Check sheet for the modelled part. Datum: model origin and axes. Units: mm. Face numbers are marked on the shaded views. A direction names the side the tool comes from. Round coordinates to 2 decimals unless told otherwise and drop trailing zeros. Order: outer loops, then holes, each group sorted by start corner. A loop starts at its lowest first (then second) coordinate and runs counter-clockwise, first axis right, second up. Notation, with made-up numbers: (34.5, 70) -> (80.5, 70) arc R9 ccw to (80.5, 77) -> close; hole circle Ø1 at (80.25, 73.25). An arc over 180 degrees is marked (long way). Answer in a Markdown table with one row per item.
```python
from build123d import *

# Parameters (mm, degrees)
F0_R     = 7.5
F1_DEPTH = 5
F2_R     = 6
F3_DEPTH = 1
F4_W     = 1.6
F4_H     = 1.2
F4_W_2   = 1.2
F4_H_2   = 1.6
F5_DEPTH = 3
F7_R     = 1.5


with BuildPart() as f1:
    # F0 (on Top) → F1 (new body)
    with BuildSketch(Plane.XY):
        Circle(F0_R)
    extrude(amount=F1_DEPTH)

    # F2 (on face) → F3 (join)
    with BuildSketch(Plane.XY.offset(5)):
        Circle(F2_R)
    extrude(amount=F3_DEPTH)

    # F4 (on face) → F5 (cut)
    with BuildSketch(Plane.XY.offset(6)):
        with Locations((0, 1.4)):
            Rectangle(F4_W, F4_H)
        with Locations((-1.4, 0)):
            Rectangle(F4_W_2, F4_H_2)
        Rectangle(F4_W, F4_H_2)
        with Locations((1.4, 0)):
            Rectangle(F4_W_2, F4_H_2)
        with Locations((0, -1.4)):
            Rectangle(F4_W, F4_H)
    extrude(amount=-F5_DEPTH, mode=Mode.SUBTRACT)

    # F7 (on Right) → F8 (revolve, cut)
    with BuildSketch(Plane.YZ):
        with Locations((-8, 2)):
            Circle(F7_R)
    revolve(axis=Axis((0, 0, 2.2380100563), (0, 0, -1)), mode=Mode.SUBTRACT)


solid = f1.part
```
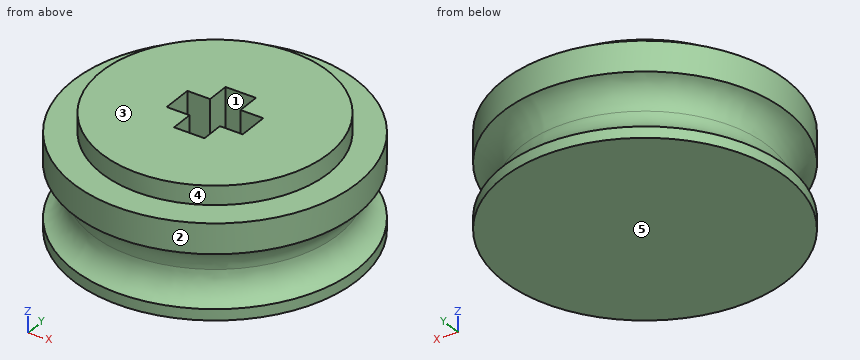
(1) Scan lines: probe 1 along X at (y, z) = (-1.25, 4.7); probe 2 along X at (y, z) = (0.75, 3.7); probe 3 along Z at (x, y) = (5.5, 3.25). Record each from-to range of solid material in increasing order. Write a range as from..to.
Solutions:
| item | result |
|---|---|
| probe 1 | -7.4..-0.8, 0.8..7.4 |
| probe 2 | -7.46..-2, 2..7.46 |
| probe 3 | 0..5 |
(2) Draft check along X on the marked faces 1, 2 and 3. Enter one of: pulls with the +X half, pulls with the -X half, needs draft (parallel to the pull), parting line crosses it, or undercut.
Solutions:
| item | result |
|---|---|
| face 1 | undercut |
| face 2 | parting line crosses it |
| face 3 | needs draft |
(3) Section check B-B on x = 0. Record the boundary of the cut face in (y, z).
Solutions:
| item | result |
|---|---|
| outline | (-7.5, 0) -> (7.5, 0) -> (7.5, 0.59) arc R1.5 cw to (7.5, 3.41) -> (7.5, 5) -> (6, 5) -> (6, 6) -> (2, 6) -> (2, 3) -> (-2, 3) -> (-2, 6) -> (-6, 6) -> (-6, 5) -> (-7.5, 5) -> (-7.5, 3.41) arc R1.5 cw to (-7.5, 0.59) -> close |
(4) Tool access check on the marked faces 4 and 5. Record the directions out of +Z, -Z, +X, -X, +Y, -Y that give a thin tool (end or side, any length) a straight path to the whole face; none if there is none.
Solutions:
| item | result |
|---|---|
| face 4 | +Z |
| face 5 | -Z, +X, -X, +Y, -Y |
(5) Depth check by flat-ended pin: pin 1 Ø1 at (x, z) = (1.5, 5) entering from -Y; pin 2 Ø3 at (y, z) = (2.5, 4.5) entering from +X; pin 3 Ø1 at (x, z) = (1.5, 4.5) entering from +Y. Enter the tip coordinate at first touch or a pass-through.
Solutions:
| item | result |
|---|---|
| pin 1 | y = -7.43 |
| pin 2 | x = 7.43 |
| pin 3 | y = 7.43 |
(6) Section check A-A on z = 4.25. Record the boundary of the cut face in (x, y).
Solutions:
| item | result |
|---|---|
| outline | circle Ø15 at (0, 0); hole (-2, -0.8) -> (-0.8, -0.8) -> (-0.8, -2) -> (0.8, -2) -> (0.8, -0.8) -> (2, -0.8) -> (2, 0.8) -> (0.8, 0.8) -> (0.8, 2) -> (-0.8, 2) -> (-0.8, 0.8) -> (-2, 0.8) -> close |
(7) Section check D-D on z = 2.8. Record the boundary of the cut face in (x, y).
Solutions:
| item | result |
|---|---|
| outline | circle Ø13.46 at (0, 0) |
